Can you work these out from the model? Positions are in its coordinate system, mm. Coordinates: 2 decimals unless noted, no trailing zeros. Loops run counter-clockwise (first coordinate to the right, second up) from the corner with the lowest first, then second, coordinate; pieces in that order, holes last.
Autodesk Inventor part; units mm, degrees
ref_plane "Work Plane1" through (-7.9612, 0, 0) normal (0, -0.866, -0.5) x (1, 0, 0)
ref_plane "YZ Plane" through (0, 0, 0) normal (1, 0, 0) x (0, 1, 0)
ref_plane "XZ Plane" through (0, 0, 0) normal (0, 1, 0) x (-1, 0, 0)
sketch "Sketch1" plane through (0, 0, 0) normal (1, 0, 0) x (0, 1, 0)
  line L0 (-4.0415, 0) -> (-2.0207, 3.5)
  line L1 (-2.0207, 3.5) -> (2.0207, 3.5)
  line L2 (2.0207, 3.5) -> (4.0415, 0)
  line L3 (4.0415, 0) -> (2.0207, -3.5)
  line L4 (2.0207, -3.5) -> (-2.0207, -3.5)
  line L5 (-2.0207, -3.5) -> (-4.0415, 0)
  point P0 (0, 0)
  point P1 (0, 0)
  dimension "d0" = 8.0829
extrude "Body" add sketch "Sketch1" along normal blind 3.2
sketch "Sketch2" plane through (0, 0, 0) normal (0, 0, 1) x (1, 0, 0)
  line L0 (0, 2.0207) -> (0, 4.0415)
  line L1 (0, 4.0415) -> (3.2, 4.0415)
  line L2 (3.2, 2.0207) -> (3.2, 4.0415)
  line L3 (-0.16, 0) -> (0.96, 0)
  line L4 (0.3126, 4.0415) -> (0, 3.5)
  line L5 (2.8874, 4.0415) -> (3.2, 3.5)
  dimension "d3" = 30
  dimension "d4" = 30
  dimension "d5" = 7
  dimension "d6" = 7
revolve "Chamfer1" cut sketch "Sketch2" angle 360 about axis through (-10, 0, 0) along (1, 0, 0)
sketch "Sketch3" plane through (3.2, 0, 0) normal (1, 0, 0) x (0, 0, -1)
  arc A0 (-1.75, -3.0311) -> (1.75, -3.0311) centre (0, 0) ccw
hole "Thread" at (3.2, 0, 0) direction (-1, 0, 0) diameter 1.221 end through all
chamfer "Chamfer2" distance 0.3789 angle 30 1 edges at (3.2, 0, 0.6105) measured on face at (3.2, 2.5226, -0.0245)
chamfer "Chamfer3" distance 0.3789 angle 30 1 edges at (0, 0, 0.6105) measured on face at (0, 2.5226, -0.0245)
ref_plane "Work Plane1" through (-7.9612, 0, 0) normal (0, -0.866, -0.5) x (1, 0, 0)
equation "\"d0\" = 1.1547 * SW"
equation "\"d1\" = KOH"
equation "\"d3\" = ANG1"
equation "\"d4\" = ANG2"
equation "\"d5\" = SW0"
equation "\"d6\" = SW01"
equation "\"d8\" = -0.5 * GD1 + 0.5 * NND"
equation "\"d40\" = -0.5 * GD1 + 0.5 * NND"
equation "\"d10\" = -0.5 * GD1 + 0.5 * NND"
equation "\"d41\" = -0.5 * GD1 + 0.5 * NND"
equation "\"ANG1\" = 30deg"
equation "\"ANG2\" = 30deg"
equation "\"NND\" = 4"
equation "\"KOH\" = 3.2"
equation "\"SW\" = 7"
equation "\"SW0\" = SW"
equation "\"SW01\" = SW"
equation "\"GUL\" = 0.541266 * PTC"
equation "\"WFT\" = 0.4"
equation "\"THREADDIA\" = 4"
equation "\"TOA\" = 30deg"
equation "\"PTC\" = 0.7"
equation "\"E0\" = 1.155 * SW"
equation "\"GAL\" = 0.541266 * PTC"
properties part number "AS 1112 - M4  Type 5" material "Steel, Mild"
Item 1: We'd pull the mould along Z, two halves only. Please class faces 1 (the face through (3.124, -3.632, -0.009)), 2 (the face through (1.58, -0.03, 0.61)), 3 (the face through (1.578, -3.045, 1.726)), 4 (the face through (3.124, -1.808, -3.15)): +Z half, -Z half, draft (parallel to the pull), parting line (faces both ways), or undercut.
Results are:
face 1: parting line
face 2: undercut
face 3: +Z half
face 4: -Z half
Item 2: Suppose I cut it at A-A, the plane x = 1.65. Please give me the cut outline in (y, z), plus the area to 3 significant figures.
Results are:
outline: (-4.04, 0) - (-2.02, -3.5) - (2.02, -3.5) - (4.04, 0) - (2.02, 3.5) - (-2.02, 3.5) - close; hole circle Ø1.22 at (0, 0)
area: 41.3 mm2
Item 3: I'm going to push a flat-ended pin straight in: P1, Ø1.5, axis at y = 3, z = -0.5, coming from the -X side. Where does the tip first touch, or does it pass through?
Results are:
P1: stops at x = 0
Item 4: I need wall thicknesses on line 1 along Z through (x, y) = (2.15, 0); line 2 along Z through (x, y) = (2.3, -0.5); line 3 along Y through (x, z) = (1.25, 3). Which ranges of each line are inside material? Lowest first, please.
Results are:
line 1: z = -3.5 to -0.61, 0.61 to 3.5
line 2: z = -3.5 to -0.35, 0.35 to 3.5
line 3: y = -2.31 to 2.31
